CAD build for the part. Positions are in the model's coordinates, mm. Face numbers are marked on the shaded views. A direction names the side the tool comes from. Coordinates: 2 decimals unless noted, no trailing zeros. Loops run counter-clockwise (first coordinate to the right, second up) from the corner with the lowest first, then second, coordinate; pieces in that order, holes last. Notation, with made-up numbers: (-8, -16) -> (28, -16) arc R17 ccw to (28, -3) -> close; hole circle Ø9 at (72, 83.5). An arc over 180 degrees is marked (long way). Return JSON: item names as keys, results as strings. Group by question number.
(1) Saw through at B-B on x = -25.5. Write the cut outline in (y, z), then the cut area to 3 significant figures.
(2) Tool access for the marked faces 5, 6 and 7: list every direction of +Z, -Z, +X, -X, +Y, -Y with a clear straight run to the whole face (end or side of a thin tool).
(3) Flat gauge pins, fed straight in: pin 1 Ø5 at (x, z) = (8, 9) entering from +Y; pin 2 Ø12 at (y, z) = (1.5, 24.5) entering from +X; pin 3 Ø1.5 at (x, y) = (24.5, 7.5) entering from +Z. Where does each tip first touch, or does it go through?
(4) Probe L1, parallel to Z at x = -22, y = 17.5; L2, parallel to X at y = -14, z = 39; L3, parallel to Y at x = 31, z = 13.5. List the from-to ranges inside material, lowest first.
(5) Mould opens along Y. For the marked faces 1, 2, 3 and 4 say: pulls with the +Y half, pulls with the -Y half, needs draft (parallel to the pull), parting line crosses it, or undercut.
(6) Saw through at C-C on y = 12. Write the cut outline in (x, z).
(7) Saw through at D-D on z = 27. Write the cut outline in (x, y), then the cut area to 3 significant figures.
(8) Saw through at A-A on y = 1. Write the cut outline in (x, z).
```python
from build123d import *

# Parameters (mm, degrees)
SKETCH1_W           = 74
SKETCH1_H           = 38
BOSS_EXTRUDE1_DEPTH = 42
SKETCH2_W           = 44
SKETCH2_H           = 6
CUT_EXTRUDE1_DEPTH  = 42
SKETCH3_W           = 16
SKETCH3_H           = 22
CUT_EXTRUDE2_DEPTH  = 74
SKETCH4_R           = 19
CUT_EXTRUDE3_DEPTH  = 15
SKETCH5_W           = 10
SKETCH5_H           = 8
CUT_EXTRUDE4_DEPTH  = 15


with BuildPart() as part:
    # Sketch1 → Boss-Extrude1 (new body)
    with BuildSketch(Plane.XY):
        Rectangle(SKETCH1_W, SKETCH1_H)
    extrude(amount=BOSS_EXTRUDE1_DEPTH)

    # Sketch2 → Cut-Extrude1 (cut)
    with BuildSketch(Plane(origin=(0, 0, 0), x_dir=(-1, 0, 0), z_dir=(0, 0, -1))):
        with Locations((0, -16)):
            Rectangle(SKETCH2_W, SKETCH2_H)
    extrude(amount=-CUT_EXTRUDE1_DEPTH, mode=Mode.SUBTRACT)

    # Sketch3 → Cut-Extrude2 (cut)
    with BuildSketch(Plane(origin=(37, 0, 0), x_dir=(0, 0, -1), z_dir=(1, 0, 0))):
        with Locations((-21, 8)):
            Rectangle(SKETCH3_W, SKETCH3_H)
    extrude(amount=-CUT_EXTRUDE2_DEPTH, mode=Mode.SUBTRACT)

    # Sketch4 → Cut-Extrude3 (cut)
    with BuildSketch(Plane(origin=(0, 19, 0), x_dir=(1, 0, 0), z_dir=(0, 1, 0))):
        with Locations((0, -21)):
            Circle(SKETCH4_R)
    extrude(amount=-CUT_EXTRUDE3_DEPTH, mode=Mode.SUBTRACT)

    # Sketch5 → Cut-Extrude4 (cut)
    with BuildSketch(Plane.XY.offset(42)):
        with Locations((-27, 10)):
            Rectangle(SKETCH5_W, SKETCH5_H)
        with Locations((27, 10)):
            Rectangle(SKETCH5_W, SKETCH5_H)
    extrude(amount=-CUT_EXTRUDE4_DEPTH, mode=Mode.SUBTRACT)


solid = part.part
```
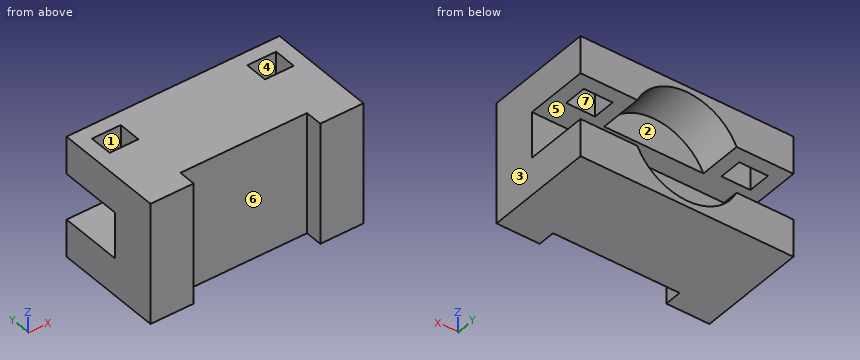
Geometry results:
{
 "1": {"outline": "(-19, 0) -> (19, 0) -> (19, 13) -> (-3, 13) -> (-3, 29) -> (6, 29) -> (6, 42) -> (-19, 42) -> close; (14, 29) -> (19, 29) -> (19, 42) -> (14, 42) -> close", "area": "1,140 mm²"},
 "2": {"face 5": "+X, -X, +Y", "face 6": "+Z, -Z, -Y", "face 7": "+Z"},
 "3": {"pin 1": "y = 4", "pin 2": "x = 37", "pin 3": "z = 13"},
 "4": {"L1": "0 to 13, 29 to 42", "L2": "-37 to -22, 22 to 37", "L3": "-19 to -3"},
 "5": {"face 1": "undercut", "face 2": "pulls with the +Y half", "face 3": "needs draft", "face 4": "undercut"},
 "6": {"outline": "(-37, 0) -> (37, 0) -> (37, 13) -> (17.23, 13) arc R19 cw to (-17.23, 13) -> (-37, 13) -> close; (-37, 29) -> (-32, 29) -> (-32, 42) -> (-37, 42) -> close; (-22, 29) -> (-17.23, 29) arc R19 cw to (17.23, 29) -> (22, 29) -> (22, 42) -> (-22, 42) -> close; (32, 29) -> (37, 29) -> (37, 42) -> (32, 42) -> close"},
 "7": {"outline": "(-37, -19) -> (-22, -19) -> (-22, -13) -> (22, -13) -> (22, -19) -> (37, -19) -> (37, -3) -> (-37, -3) -> close", "area": "920 mm²"},
 "8": {"outline": "(-37, 0) -> (37, 0) -> (37, 13) -> (-37, 13) -> close; (-37, 29) -> (37, 29) -> (37, 42) -> (-37, 42) -> close"}
}
